```python
from build123d import *

# Parameters (mm, degrees)
CROQUIS1_W              = 19.5
CROQUIS1_H              = 19.5
SALIENTE_EXTRUIR1_DEPTH = 11
CHAFL_N1_SIZE           = 2
SALIENTE_EXTRUIR2_DEPTH = 9
CROQUIS3_R              = 7.75
SALIENTE_EXTRUIR3_DEPTH = 7.2
CORTAR_EXTRUIR1_DEPTH   = 3.2
CROQUIS5_R              = 7
SALIENTE_EXTRUIR4_DEPTH = 1.7
C_PULA1_FACE_RADIUS     = 7
C_PULA1_HEIGHT          = 2.5
REDONDEO1_R             = 1


with BuildPart() as part:
    # Croquis1 → Saliente-Extruir1 (new body)
    with BuildSketch(Plane(origin=(0, 0, 0), x_dir=(1, 0, 0), z_dir=(0, 1, 0))):
        Rectangle(CROQUIS1_W, CROQUIS1_H)
    extrude(amount=SALIENTE_EXTRUIR1_DEPTH)

    # Chaflán1
    chafl_n1_edges = [part.edges().sort_by_distance(p)[0] for p in [
        (-9.75, 11, 0),
        (0, 11, 9.75),
        (9.75, 11, 0),
        (0, 11, -9.75),
    ]]
    chamfer(chafl_n1_edges, length=CHAFL_N1_SIZE)

    # Croquis2 → Saliente-Extruir2 (add)
    with BuildSketch(Plane(origin=(9.75, 0, 0), x_dir=(0, 0, -1), z_dir=(1, 0, 0))):
        with BuildLine():
            ThreePointArc((-0.6, 9), (-0.447213595, 10.694427191), (1, 9.8))
            ThreePointArc((1, 9.8), (0.894427191, 9.352786405), (0.6, 9))
            Line((0.6, 9), (2.891366459, 9))
            ThreePointArc((2.891366459, 9), (2.972717559, 9.396328956), (3, 9.8))
            ThreePointArc((3, 9.8), (-0.403671044, 12.772717559), (-2.891366459, 9))
            Line((-2.891366459, 9), (-0.6, 9))
        make_face()
        with BuildLine():
            ThreePointArc((0.6, 9), (0, 8.8), (-0.6, 9))
            Line((-0.6, 9), (-2.891366459, 9))
            ThreePointArc((-2.891366459, 9), (0, 6.8), (2.891366459, 9))
            Line((2.891366459, 9), (0.6, 9))
        make_face()
    extrude(amount=-SALIENTE_EXTRUIR2_DEPTH)

    # Croquis3 → Saliente-Extruir3 (add)
    with BuildSketch(Plane(origin=(0, 11, 0), x_dir=(1, 0, 0), z_dir=(0, 1, 0))):
        with Locations(Location((0, 0, 0), (0, 0, 270))):
            Circle(CROQUIS3_R)
    extrude(amount=SALIENTE_EXTRUIR3_DEPTH)

    # Croquis4 → Cortar-Extruir1 (cut)
    with BuildSketch(Plane(origin=(9.75, 0, 0), x_dir=(0, 0, -1), z_dir=(1, 0, 0))):
        with BuildLine():
            Line((-0.6, 9), (0.6, 9))
            ThreePointArc((0.6, 9), (0, 10.8), (-0.6, 9))
        make_face()
    extrude(amount=-CORTAR_EXTRUIR1_DEPTH, mode=Mode.SUBTRACT)

    # Croquis5 → Saliente-Extruir4 (add)
    with BuildSketch(Plane(origin=(0, 18.2, 0), x_dir=(1, 0, 0), z_dir=(0, 1, 0))):
        with Locations(Location((0, 0, 0), (0, 0, 270))):
            Circle(CROQUIS5_R)
    extrude(amount=SALIENTE_EXTRUIR4_DEPTH)

    # Cúpula1: a dome of height H over a round flat face of radius A is a cap of a sphere of radius (A * A + H * H) / (2 * H)
    c_pula1_r = (C_PULA1_FACE_RADIUS * C_PULA1_FACE_RADIUS + C_PULA1_HEIGHT * C_PULA1_HEIGHT) / (2 * C_PULA1_HEIGHT)
    c_pula1_base = Plane((0, 19.9, 0), z_dir=(0, 1, 0))
    with Locations(c_pula1_base.offset(C_PULA1_HEIGHT - c_pula1_r)):
        c_pula1_ball = Sphere(c_pula1_r, mode=Mode.PRIVATE)
    add(split(c_pula1_ball, bisect_by=c_pula1_base, keep=Keep.TOP, mode=Mode.PRIVATE))

    # Redondeo1
    redondeo1_edges = [part.edges().sort_by_distance(p)[0] for p in [
        (0, 19.9, -7),
    ]]
    fillet(redondeo1_edges, radius=REDONDEO1_R)


solid = part.part
```
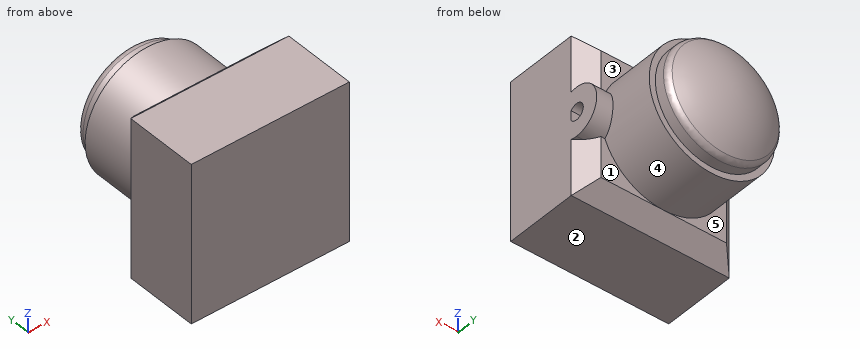
Part model, mm, in its own coordinate system. Face numbers are marked on the shaded views. A direction names the side the tool comes from. Coordinates: 2 decimals unless noted, no trailing zeros. Order: outer loops, then holes, each group sorted by start corner. A loop starts at its lowest first (then second) coordinate and runs counter-clockwise, first axis right, second up. Notation, with made-up numbers: (29.5, 25.25) -> (54.5, 25.25) arc R11 cw to (54.5, 36.25) -> close; hole circle Ø2 at (68, -24.75). An arc over 180 degrees is marked (long way). Put each result on its own line as item: value. Start each with the question number.
(1) Which spindle directions (+Z, -Z, +X, -X, +Y, -Y) get a long thin tool onto all of the face, cutting with end or side? Do the marked faces 1, 2, 3, 4 and 5. Say none if no direction does.
(2) Probe line 1 along Y through (x, z) = (8.65, 0); line 2 along Z through (x, y) = (9.05, 9.8); line 3 along Y through (x, z) = (7.45, 0). List the from-to ranges inside material, lowest first. Write a range as [from, to].
(3) Band-saw the part on B-B (y = 14.25). Give the cut face in (x, z).
(4) Pin check, flat tips, straight feed: pin 1 Ø0.9 at (y, z) = (9.5, 0) entering from +X; pin 2 Ø6 at (x, z) = (-4, 5.5) entering from +Y; pin 3 Ø2 at (x, y) = (-6, 20) entering from -Z. Stop position of each tip, or through.
(5) Band-saw the part on A-A (y = 18.75). Give the cut face in (x, z).
Determined:
1. face 1: -Z, +X, +Y
1. face 2: -Z, +X, -X, +Y, -Y
1. face 3: +Z, +X, +Y
1. face 4: +Y
1. face 5: -Z, -X, +Y
2. line 1: y = [0, 9], [10.8, 12.8]
2. line 2: z = [-3, -1], [1, 3]
2. line 3: y = [0, 9], [10.8, 18.2]
3. outline: circle Ø15.5 at (0, 0)
4. pin 1: stops at x = 6.55
4. pin 2: stops at y = 21.73
4. pin 3: stops at z = -4.79
5. outline: circle Ø14 at (0, 0)
